Build history of the part. All positions in model axes, mm. A direction names the side the tool comes from. Round coordinates to 2 decimals unless told otherwise and drop trailing zeros. Write each loop counter-clockwise with the first axis right and the second up, starting at its lowest first coordinate (ties: lowest second). Pieces come first, ordered by that corner, then holes. Notation, with made-up numbers: M -34,-19.75 L -30,-19.75 A10 cw -30,-13.75 Z; hole C 57,86 d7. An arc over 180 degrees is marked long. Use a Markdown table: item, result.
from build123d import *

# Parameters (mm, degrees)
SKETCH1_W           = 57
SKETCH1_H           = 48
SKETCH1_W_2         = 2
SKETCH1_H_2         = 20
SKETCH1_R           = 2.125
BOSS_EXTRUDE1_DEPTH = 7
SKETCH1_3_W         = 20.1
SKETCH1_3_H         = 20
BOSS_EXTRUDE2_DEPTH = 2


with BuildPart() as part:
    # Sketch1 → Boss-Extrude1 (new body)
    # profile 1 of 3: a face of its own
    with BuildSketch(Plane(origin=(0, 0, 0), x_dir=(1, 0, 0), z_dir=(0, 1, 0))):
        Polygon((32.185274303, -10), (32.185274303, 10), (32.185274303, 27.483916231), (-32.185274303, 27.483916231), (-32.185274303, -27.483916231), (32.185274303, -27.483916231), align=None)
        with Locations((0, -0.016083769)):
            Rectangle(SKETCH1_W, SKETCH1_H, mode=Mode.SUBTRACT)
    # profile 2 of 3: a face of its own
    with BuildSketch(Plane(origin=(0, 0, 0), x_dir=(1, 0, 0), z_dir=(0, 1, 0))):
        with Locations((53.285274303, 0)):
            Rectangle(SKETCH1_W_2, SKETCH1_H_2)
    # profile 3 of 3: a face of its own
    with BuildSketch(Plane(origin=(0, 0, 0), x_dir=(1, 0, 0), z_dir=(0, 1, 0))):
        with Locations((0, -0.016083769)):
            Rectangle(SKETCH1_W, SKETCH1_H)
        with Locations(Location((25.94552801, -21.035, 0), (0, 0, 270))):
            Circle(SKETCH1_R, mode=Mode.SUBTRACT)
        with Locations(Location((-22.09447199, -21.035, 0), (0, 0, 270))):
            Circle(SKETCH1_R, mode=Mode.SUBTRACT)
        with Locations(Location((-22.09447199, 21.035, 0), (0, 0, 270))):
            Circle(SKETCH1_R, mode=Mode.SUBTRACT)
        with Locations(Location((25.94552801, 21.035, 0), (0, 0, 270))):
            Circle(SKETCH1_R, mode=Mode.SUBTRACT)
    extrude(amount=BOSS_EXTRUDE1_DEPTH)

    # Sketch1_3 → Boss-Extrude2 (add)
    with BuildSketch(Plane(origin=(0, 0, 0), x_dir=(1, 0, 0), z_dir=(0, 1, 0))):
        with Locations((42.235274303, 0)):
            Rectangle(SKETCH1_3_W, SKETCH1_3_H)
    extrude(amount=BOSS_EXTRUDE2_DEPTH)


solid = part.part
Q1. Cut at C-C on x = 38.5. Give the cut face in (y, z).
Response values:
| item | result |
|---|---|
| outline | M 0,-10 L 2,-10 L 2,10 L 0,10 Z |
Q2. Cut at B-B on z = 3. Give the cut face in (x, y), and give its area (3 significant figures).
Response values:
| item | result |
|---|---|
| outline | M -32.19,0 L 54.29,0 L 54.29,7 L 52.29,7 L 52.29,2 L 32.19,2 L 32.19,7 L -32.19,7 Z |
| area | 505 mm2 |
Q3. Two-plate mould, pull along X, no slides. Class faces 1 (the flat face through (52.285, 4, 0)), 2 (the flat face through (0, 3, 27.484)), 3 (the flat face through (32.185, 3, 0)), 4 (the flat face through (54.285, 3, 0)): +X half, -X half, draft (parallel to the pull), parting line (faces both ways), or undercut.
Response values:
| item | result |
|---|---|
| face 1 | undercut |
| face 2 | draft |
| face 3 | undercut |
| face 4 | +X half |
Q4. Cut at A-A on y = 4. Give the cut face in (x, z) (3 decimals).
Response values:
| item | result |
|---|---|
| outline | M -32.185,-27.484 L 32.185,-27.484 L 32.185,27.484 L -32.185,27.484 Z; M 52.285,-10 L 54.285,-10 L 54.285,10 L 52.285,10 Z; hole C -22.094,-21.035 d4.25; hole C -22.094,21.035 d4.25; hole C 25.946,-21.035 d4.25; hole C 25.946,21.035 d4.25 |
Q5. Which spindle directions (+Z, -Z, +X, -X, +Y, -Y) get a long thin tool onto all of the face, cutting with end or side? Do faces 5 (the cylindrical face through (28.052, 3.451, -21.312)), 6 (the flat face through (46, 1, 10)), 7 (the flat face through (42, 2, 0)), 8 (the flat face through (46, 1, -10)). Say none if no direction does.
Response values:
| item | result |
|---|---|
| face 5 | +Y, -Y |
| face 6 | +Z, +X, +Y, -Y |
| face 7 | +Z, -Z, +Y |
| face 8 | -Z, +X, +Y, -Y |
Q6. Drop flat-ended pins along their axis: P1, Ø2.5, axis at x = 25.95, z = -21.04, coming from the -Y side; P2, Ø1.5, axis at y = 4.5, z = 12.5, coming from the +X side. Give the stop position or say it passes through.
Response values:
| item | result |
|---|---|
| P1 | passes through |
| P2 | stops at x = 32.19 |
Q7. Drill centre lines: L1, parallel to Z at x = -24, y = 4.5; L2, parallel to Z at x = -21.5, y = 5.5; L3, parallel to X at y = 5, z = -4. Where is each one in solid material? Low to high.
Response values:
| item | result |
|---|---|
| L1 | z = -27.48 to -21.98, -20.09 to 20.09, 21.98 to 27.48 |
| L2 | z = -27.48 to -23.08, -18.99 to 18.99, 23.08 to 27.48 |
| L3 | x = -32.19 to 32.19, 52.29 to 54.29 |
Q8. Cut at D-D on z = 12.5. Give the cut face in (x, y).
Response values:
| item | result |
|---|---|
| outline | M -32.19,0 L 32.19,0 L 32.19,7 L -32.19,7 Z |
